Check sheet for the modelled part. Datum: model origin and axes. Units: mm. A direction names the side the tool comes from. Give positions to 0.01 mm unless a question says otherwise; leave off trailing zeros. Write each loop counter-clockwise with the first axis right and the second up, starting at its lowest first coordinate (ties: lowest second). Pieces come first, ordered by that corner, then holes. Notation, with made-up numbers: M 31.5,-40 L 90.5,-40 A25 ccw 90.5,-26 Z; hole C -2,32 d4. An arc over 180 degrees is marked long. Write item = value, one per line. Start each with the question number.
1) Access from +Z, -Z, +X, -X, +Y, -Y to the whole of each face (thin tool, end or side, straight path). Record for faces 1 (the cylindrical face through (15.57, 39.07, 14)), 2 (the flat face through (-21.15, 22, 0)).
2) Cross-section at C-C, the plane y = 41. Record the cut outline in (x, z), plus the area to 3 significant figures.
3) Cross-section at B-B, the plane x = 0. Record the cut outline in (y, z), plus the area to 3 significant figures.
4) Mould release check, pull along X, two halves, no side actions. Record for faces 3 (the cylindrical face through (-2.44, 54.35, -0.54)), 4 (the flat face through (0, 22, 21.15)), 5 (the flat face through (-15, 34, -16)), 6 (the flat face through (18.2, 21.7, -18.1)): released by +X, released by -X, zero draft, split by the parting line, or undercut.
5) Cross-section at D-D, the plane y = 23.5. Record the cut outline in (x, z).
6) Go/stop test with flat-tipped pins: pin 1 (3.5 mm diameter, centred on x = -16, z = -15, fed in from +Y); pin 2 (1.5 mm diameter, centred on x = -16, z = 15.5, fed in from +Y). Record where each tip stops, or that it passes through.
7) Cross-section at A-A, the plane z = 0. Record the cut outline in (x, y).
8) Scan lines: line 1 along Z through (x, y) = (15, 39); line 2 along X through (y, z) = (36.5, -14.5). Record each from-to range of solid material in increasing order. Write a range as [from, to].
```python
from build123d import *

# Parameters (mm, degrees)
SKETCH1_W           = 42.3
SKETCH1_H           = 42.3
SKETCH1_R           = 2.5
BOSS_EXTRUDE1_DEPTH = 44
SKETCH1_3_R         = 2.5
BOSS_EXTRUDE2_DEPTH = 66
CHAMFER1_SIZE       = 6
CHAMFER2_SIZE       = 1
SKETCH2_R           = 1.5
CUT_EXTRUDE1_DEPTH  = 10


with BuildPart() as part:
    # Sketch1 → Boss-Extrude1 (new body)
    with BuildSketch(Plane(origin=(0, 0, 0), x_dir=(1, 0, 0), z_dir=(0, 1, 0))):
        Rectangle(SKETCH1_W, SKETCH1_H)
        Circle(SKETCH1_R, mode=Mode.SUBTRACT)
        Circle(SKETCH1_R)
    extrude(amount=BOSS_EXTRUDE1_DEPTH)

    # Sketch1_3 → Boss-Extrude2 (add)
    with BuildSketch(Plane(origin=(0, 0, 0), x_dir=(1, 0, 0), z_dir=(0, 1, 0))):
        with Locations(Location((0, 0, 0), (0, 0, 270))):  # turned: the seam where the file's is
            Circle(SKETCH1_3_R)
    extrude(amount=BOSS_EXTRUDE2_DEPTH)

    # Chamfer1
    chamfer1_edges = [part.edges().sort_by_distance(p)[0] for p in [
        (21.15, 22, 21.15),
        (-21.15, 22, 21.15),
        (-21.15, 22, -21.15),
        (21.15, 22, -21.15),
    ]]
    chamfer(chamfer1_edges, length=CHAMFER1_SIZE)

    # Chamfer2
    chamfer2_edges = [part.edges().sort_by_distance(p)[0] for p in [
        (0, 66, -2.5),
    ]]
    chamfer(chamfer2_edges, length=CHAMFER2_SIZE)

    # Sketch2 → Cut-Extrude1 (cut)
    with BuildSketch(Plane(origin=(0, 44, 0), x_dir=(1, 0, 0), z_dir=(0, 1, 0))):
        with Locations(Location((-15.5, 15.5, 0), (0, 0, 270))):  # turned: the seam where the file's is
            Circle(SKETCH2_R)
        with Locations(Location((15.5, 15.5, 0), (0, 0, 270))):  # turned: the seam where the file's is
            Circle(SKETCH2_R)
        with Locations(Location((15.5, -15.5, 0), (0, 0, 270))):  # turned: the seam where the file's is
            Circle(SKETCH2_R)
        with Locations(Location((-15.5, -15.5, 0), (0, 0, 270))):  # turned: the seam where the file's is
            Circle(SKETCH2_R)
    extrude(amount=-CUT_EXTRUDE1_DEPTH, mode=Mode.SUBTRACT)


solid = part.part
```
Reply:
q1.face_1 = +Y
q1.face_2 = +Z, -Z, -X, +Y, -Y
q2.outline = M -21.15,-15.15 L -15.15,-21.15 L 15.15,-21.15 L 21.15,-15.15 L 21.15,15.15 L 15.15,21.15 L -15.15,21.15 L -21.15,15.15 Z; hole C -15.5,-15.5 d3; hole C -15.5,15.5 d3; hole C 15.5,-15.5 d3; hole C 15.5,15.5 d3
q2.area = 1,690 mm2
q3.outline = M 0,-21.15 L 44,-21.15 L 44,-2.5 L 65,-2.5 L 66,-1.5 L 66,1.5 L 65,2.5 L 44,2.5 L 44,21.15 L 0,21.15 Z
q3.area = 1,970 mm2
q4.face_3 = split by the parting line
q4.face_4 = zero draft
q4.face_5 = undercut
q4.face_6 = released by +X
q5.outline = M -21.15,-15.15 L -15.15,-21.15 L 15.15,-21.15 L 21.15,-15.15 L 21.15,15.15 L 15.15,21.15 L -15.15,21.15 L -21.15,15.15 Z
q6.pin_1 = 44
q6.pin_2 = 34
q7.outline = M -21.15,0 L 21.15,0 L 21.15,44 L 2.5,44 L 2.5,65 L 1.5,66 L -1.5,66 L -2.5,65 L -2.5,44 L -21.15,44 Z
q8.line_1 = [-21.15, -16.91], [-14.09, 14.09], [16.91, 21.15]
q8.line_2 = [-21.15, -16.62], [-14.38, 14.38], [16.62, 21.15]
